Could you check a few things on this model? Use its own coordinates, in mm. Face numbers are marked on the shaded views. A direction names the side the tool comes from. Coordinates: 2 decimals unless noted, no trailing zeros. Loops run counter-clockwise (first coordinate to the right, second up) from the corner with the lowest first, then second, coordinate; pieces in that order, holes last. Notation, with made-up numbers: (61.25, 75.25) - (113.25, 75.25) arc R24 cw to (113.25, 111.25) - close; hole circle Ø1 at (23, -36). An arc over 180 degrees is marked (long way). Use CSV: the item, a comma, the result in double quotes.
from build123d import *

# Parameters (mm, degrees)
F1_DEPTH = 50.8


with BuildPart() as f1:
    # F0 (on Front) → F1 (new body)
    with BuildSketch(Plane.XZ):
        Polygon((-31.75, -19.05), (0, -19.05), (31.75, -19.05), (31.75, 63.5), (82.55, 63.5), (82.55, 88.9), (-82.55, 88.9), (-82.55, 63.5), (-31.75, 63.5), align=None)
        with BuildLine():
            ThreePointArc((0, 9.652), (6.824994652, 6.824994652), (9.652, 0))
            ThreePointArc((9.652, 0), (-6.824994652, -6.824994652), (0, 9.652))
        make_face(mode=Mode.SUBTRACT)
        with BuildLine():
            ThreePointArc((6.35, 69.85), (4.4901280605, 65.3598719395), (0, 63.5))
            ThreePointArc((0, 63.5), (-4.4901280605, 74.3401280605), (6.35, 69.85))
        make_face(mode=Mode.SUBTRACT)
    extrude(amount=F1_DEPTH)


solid = f1.part
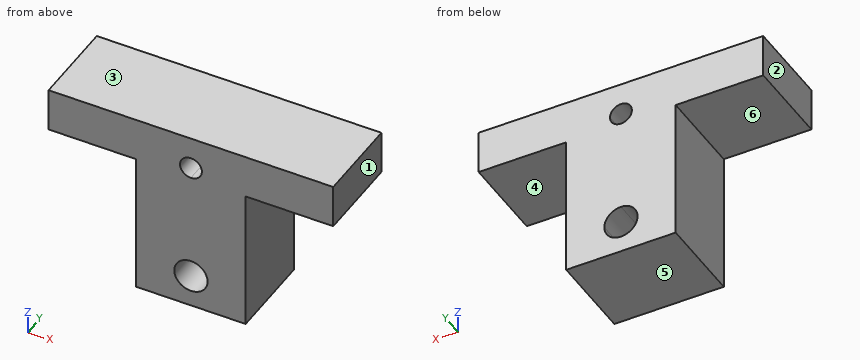
(1) Suppose I cut it at A-A (y = -24). Write out the boundary of the cut face in (x, z), plus the area to 3 significant figures.
Computed:
outline,"(-82.55, 63.5) - (-31.75, 63.5) - (-31.75, -19.05) - (31.75, -19.05) - (31.75, 63.5) - (82.55, 63.5) - (82.55, 88.9) - (-82.55, 88.9) - close; hole circle Ø19.3 at (0, 0); hole circle Ø12.7 at (0, 69.85)"
area,"9,020 mm²"
(2) Which directions (+Z, -Z, +X, -X, +Y, -Y) give clear straight access to the entire face, cutting with the end or side of a thin tool? Please do the marked faces 4, 5 and 6.
Computed:
face 4,"-Z, +X, +Y, -Y"
face 5,"-Z, +X, -X, +Y, -Y"
face 6,"-Z, -X, +Y, -Y"
(3) Suppose I cut it at D-D (z = 32). Write out the boundary of the cut face in (x, y).
Computed:
outline,"(-31.75, -50.8) - (31.75, -50.8) - (31.75, 0) - (-31.75, 0) - close"
(4) Thinking about a two-plate mould opening in X: for the marked faces 1, 2 and 3, which applies, +X half, -X half, draft (parallel to the pull), parting line (faces both ways), or undercut?
Computed:
face 1,"+X half"
face 2,"-X half"
face 3,"draft"
(5) Will these pins go through, and if not, where does the flat tip stop? pin 1 (4 mm diameter, centred on y = -40, z = 41, fed in from +X); pin 2 (15 mm diameter, centred on y = -17.5, z = 36.5, fed in from -X); pin 3 (2 mm diameter, centred on x = 44.5, y = -33, fed in from -Z).
Computed:
pin 1,"stops at x = 31.75"
pin 2,"stops at x = -31.75"
pin 3,"stops at z = 63.5"
(6) Suppose I cut it at B-B (z = -7). Write out the boundary of the cut face in (x, y).
Computed:
outline,"(-31.75, -50.8) - (-6.65, -50.8) - (-6.65, 0) - (-31.75, 0) - close; (6.65, -50.8) - (31.75, -50.8) - (31.75, 0) - (6.65, 0) - close"
(7) Please list where these lines run through material, in increasing order: line 1 (Z direction, x = 0, y = -13); line 2 (Z direction, x = 72, y = -14); line 3 (X direction, y = -34.5, z = 26.5).
Computed:
line 1,"z = -19.05 to -9.65, 9.65 to 63.5, 76.2 to 88.9"
line 2,"z = 63.5 to 88.9"
line 3,"x = -31.75 to 31.75"
(8) Suppose I cut it at C-C (x = -49). Write out the boundary of the cut face in (y, z).
Computed:
outline,"(-50.8, 63.5) - (0, 63.5) - (0, 88.9) - (-50.8, 88.9) - close"
